```python
from build123d import *

# Parameters (mm, degrees)
F0_W      = 203.2
F0_H      = 101.6
F1_DEPTH  = 101.6
F2_W      = 203.2
F2_H      = 50.8
F3_DEPTH  = 50.8
F4_W      = 50.8
F4_H      = 50.8
F5_DEPTH  = 76.2
F6_W      = 50.8
F6_H      = 50.8
F7_DEPTH  = 76.2
F8_R      = 25.4
F9_R      = 25.4
F12_D     = 6.35
F11_R     = 12.7
F13_DEPTH = 101.6
F14_R     = 12.7
F14_R_2   = 3.175
F15_DEPTH = 101.6


with BuildPart() as f1:
    # F0 (on Front) → F1 (new body)
    with BuildSketch(Plane.XZ):
        with Locations((-14.2620336264, 18.2871496212)):
            Rectangle(F0_W, F0_H)
    extrude(amount=F1_DEPTH)

    # F2 (on face) → F3 (cut)
    with BuildSketch(Plane.XZ.offset(101.6)):
        with Locations((-14.2620336264, -7.1128503788)):
            Rectangle(F2_W, F2_H)
    extrude(amount=-F3_DEPTH, mode=Mode.SUBTRACT)

    # F4 (on face) → F5 (cut)
    with BuildSketch(Plane(origin=(0, 0, -32.5128503788), x_dir=(1, 0, 0), z_dir=(0, 0, -1))):
        with Locations((61.9379663736, 25.4)):
            Rectangle(F4_W, F4_H)
    extrude(amount=-F5_DEPTH, mode=Mode.SUBTRACT)

    # F6 (on face) → F7 (cut)
    with BuildSketch(Plane(origin=(0, 0, -32.5128503788), x_dir=(1, 0, 0), z_dir=(0, 0, -1))):
        with Locations((-90.4620336264, 25.4)):
            Rectangle(F6_W, F6_H)
    extrude(amount=-F7_DEPTH, mode=Mode.SUBTRACT)

    # F8
    f8_edges = [f1.edges().sort_by_distance(p)[0] for p in [
        (87.337966, -101.6, 43.68715),
    ]]
    fillet(f8_edges, radius=F8_R)

    # F9
    f9_edges = [f1.edges().sort_by_distance(p)[0] for p in [
        (-115.862034, -101.6, 43.68715),
    ]]
    fillet(f9_edges, radius=F9_R)

    # F12 (through all)
    with Locations(Plane(origin=(0, 0, 18.2871496212), x_dir=(1, 0, 0), z_dir=(0, 0, -1))):
        with Locations((-94.1294133663, 77.4258524179)):
            Hole(F12_D / 2)

    # F11 (on face) → F13 (cut)
    with BuildSketch(Plane(origin=(0, 0, 18.2871496212), x_dir=(1, 0, 0), z_dir=(0, 0, -1))):
        with Locations((60.9464161098, 77.4258524179)):
            Circle(F11_R)
    extrude(amount=-F13_DEPTH, mode=Mode.SUBTRACT)

    # F14 (on face) → F15 (cut)
    with BuildSketch(Plane(origin=(0, 0, 18.2871496212), x_dir=(1, 0, 0), z_dir=(0, 0, -1))):
        with Locations((-94.1294133663, 77.4258524179)):
            Circle(F14_R)
        with Locations((-94.1294133663, 77.4258524179)):
            Circle(F14_R_2, mode=Mode.SUBTRACT)
    extrude(amount=-F15_DEPTH, mode=Mode.SUBTRACT)


solid = f1.part
```
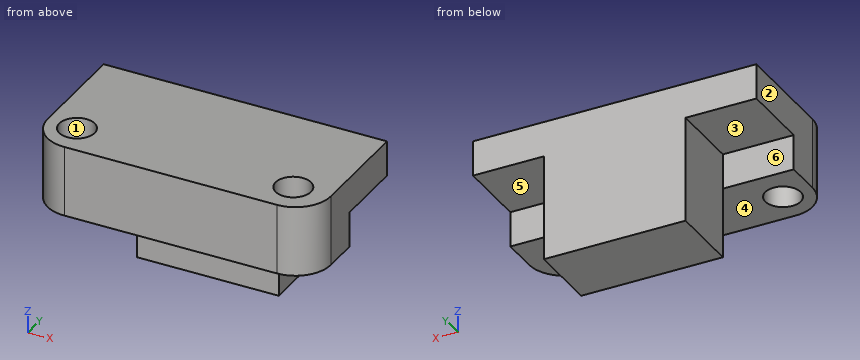
Can you work these out from the model? Positions are in its coordinate system, mm. Face numbers are marked on the shaded views. A direction names the side the tool comes from. Give positions to 0.01 mm unless a question says otherwise; leave off trailing zeros. Write each loop counter-clockwise with the first axis right and the second up, starting at its lowest first coordinate (ties: lowest second). Pieces come first, ordered by that corner, then holes. Notation, with made-up numbers: (-11, -23) - (16, -23) arc R24 cw to (16, 8) - close; hole circle Ø5 at (58, 43.5). An arc over 180 degrees is marked (long way). Write item = value, one per line. Start each with the question number.
1. On a 3-axis mill with a long thin cutter (end or side, diameter ignored), from which of +Z, -Z, +X, -X, +Y, -Y can I reach the whole of each face in a straight line? I mean the marked faces 4, 5 and 6. Say none if no direction works.
2. Imagine slicing it at C-C (z = 51). Please give me the cut outline in (x, y), and give its area (3 significant figures).
3. Imagine slicing it at A-A (y = -80.5). Please give me the cut outline in (x, z), and give its area (3 significant figures).
4. Imagine slicing it at B-B (x = 70.5). Please give me the cut outline in (y, z).
5. Please list where these lines run through material, in increasing order: line 1 (Y direction, x = 29, z = 16); line 2 (Z direction, x = -80, y = -38); line 3 (Z direction, x = -55.5, y = -70).
6. Imagine slicing it at D-D (y = -22.5). Please give me the cut outline in (x, z).
7. For pin 1 (10 mm diameter, centred on x = -10, z = 19.5, fed in from +Y); pin 2 (10 mm diameter, centred on x = -32.5, z = 9.5, fed in from -Y); pin 3 (12.5 mm diameter, centred on x = -96, z = 33, fed in from +Y), each with a flat end and sliding along its axis, tell me the tip position at first contact or that it passes through.
8. Thinking about a two-plate mould opening in X: for the marked faces 1, 2 and 3, which applies, released by +X, released by -X, zero draft, split by the parting line, or undercut?
Worked answers:
q1.face_4 = -Z, +X, -X, -Y
q1.face_5 = -Z, +X, +Y
q1.face_6 = -Z, -X, +Y
q2.outline = (-115.86, -76.2) arc R25.4 ccw to (-90.46, -101.6) - (61.94, -101.6) arc R25.4 ccw to (87.34, -76.2) - (87.34, 0) - (-115.86, 0) - close; hole circle Ø25.4 at (-94.13, -77.43); hole circle Ø25.4 at (60.95, -77.43)
q2.area = 19,400 mm2
q3.outline = (-115.5, 18.29) - (-106.45, 18.29) - (-106.45, 69.09) - (-115.5, 69.09) - close; (-81.81, 18.29) - (48.62, 18.29) - (48.62, 69.09) - (-81.81, 69.09) - close; (73.27, 18.29) - (86.97, 18.29) - (86.97, 69.09) - (73.27, 69.09) - close
q3.area = 7,780 mm2
q4.outline = (-100.11, 18.29) - (-85.79, 18.29) - (-85.79, 69.09) - (-100.11, 69.09) - close; (-69.06, 18.29) - (-50.8, 18.29) - (-50.8, 43.69) - (0, 43.69) - (0, 69.09) - (-69.06, 69.09) - close
q5.line_1 = -50.8 to 0
q5.line_2 = 43.69 to 69.09
q5.line_3 = 18.29 to 69.09
q6.outline = (-115.86, 43.69) - (-65.06, 43.69) - (-65.06, -32.51) - (36.54, -32.51) - (36.54, 43.69) - (87.34, 43.69) - (87.34, 69.09) - (-115.86, 69.09) - close
q7.pin_1 = 0
q7.pin_2 = -50.8
q7.pin_3 = -50.8
q8.face_1 = undercut
q8.face_2 = released by -X
q8.face_3 = zero draft
